Verification items for this drawing (mm, ordinates from the low corner). Round coordinates to 2 decimals unless told otherwise and drop trailing zeros. Loops run counter-clockwise (first coordinate to the right, second up) from the corner with the lowest first, then second, coordinate; pieces in that order, holes last. Notation, with made-up numbers: (-17, 52) - (42, 52) arc R16 cw to (42, 57) - close; hole circle Ø8 at (10.25, 83). An arc over 180 degrees is marked (long way). Answer in a Markdown table with one row per item. Add a question column.
(1) Cross-section at D-D on x = 1.15. Enter the section's corners in (y, z), then the cut area to 3 significant figures.
(2) Cross-section at B-B on z = 24. Enter the section's corners in (x, y).
(3) Cross-section at A-A on x = 2.9. Enter the section's corners in (y, z), then the cut area to 3 significant figures.
(4) Cross-section at C-C on y = 15.5. Enter the section's corners in (x, z).
(5) Thickness scan on line 1 along Y through (x, z) = (3.5, 6.5); line 2 along X through (y, z) = (5.5, 32); line 3 along Z through (x, y) = (2.2, 15.5). Record the ranges inside material, lowest first.
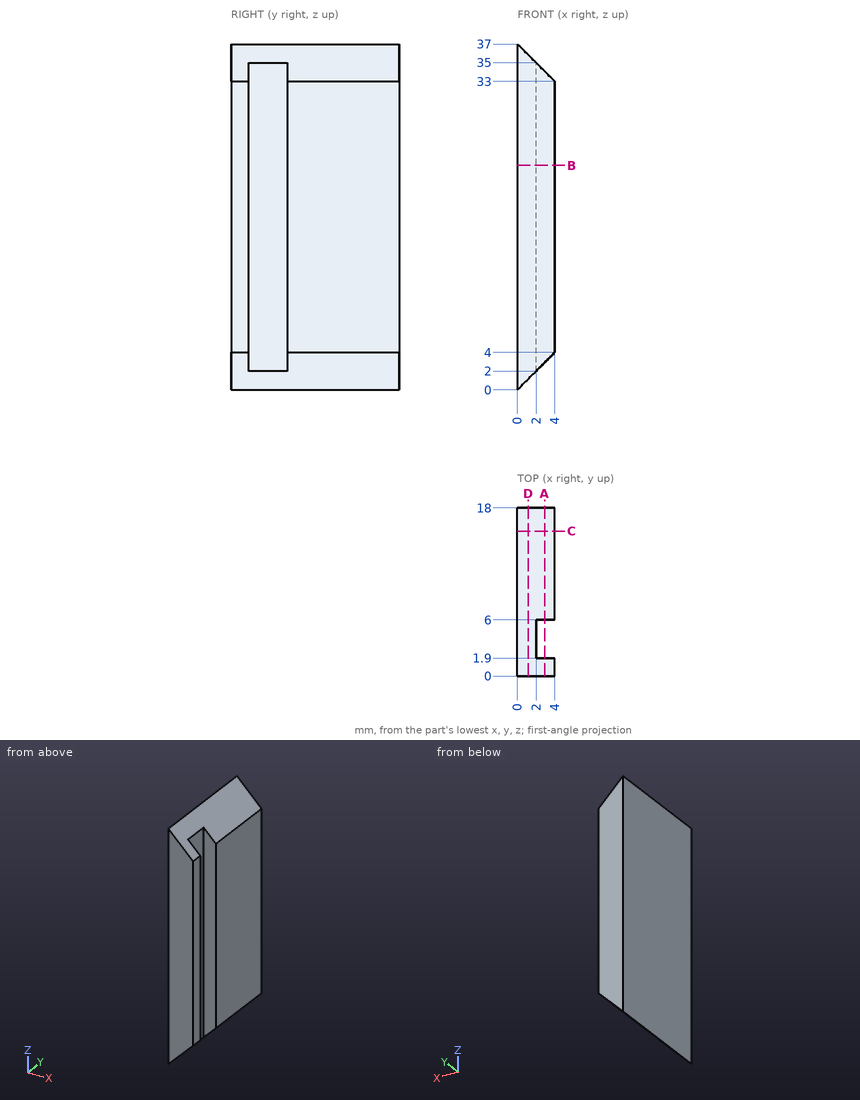
Answers:
| question | item | result |
|---|---|---|
| 1 | outline | (0, 1.15) - (18, 1.15) - (18, 35.85) - (0, 35.85) - close |
| 1 | area | 625 mm^2 |
| 2 | outline | (0, 0) - (4, 0) - (4, 1.9) - (2, 1.9) - (2, 6) - (4, 6) - (4, 18) - (0, 18) - close |
| 3 | outline | (0, 2.9) - (1.9, 2.9) - (1.9, 34.1) - (0, 34.1) - close; (6, 2.9) - (18, 2.9) - (18, 34.1) - (6, 34.1) - close |
| 3 | area | 434 mm^2 |
| 4 | outline | (0, 0) - (4, 4) - (4, 33) - (0, 37) - close |
| 5 | line 1 | y = 0 to 1.9, 6 to 18 |
| 5 | line 2 | x = 0 to 2 |
| 5 | line 3 | z = 2.2 to 34.8 |
